The model under review builds one solid part; all positions refer to its coordinate system, in mm. Face numbers are marked on the shaded views. A direction names the side the tool comes from. Coordinates: 2 decimals unless noted, no trailing zeros. Write each loop counter-clockwise with the first axis right and the second up, starting at its lowest first coordinate (ties: lowest second). Pieces come first, ordered by that corner, then holes. Notation, with made-up numbers: M -15.5,3 L 12.5,3 A9 cw 12.5,15 Z; hole C 46.25,4.25 d6. An arc over 180 degrees is marked long. Answer as a JSON object with one key per item and string values.
```python
from build123d import *

# Parameters (mm, degrees)
SKETCH1_W                 = 32.5
SKETCH1_H                 = 42
BOSS_EXTRUDE2_DEPTH       = 5
F_2_56_TAPPED_HOLE1_D     = 1.778
F_2_56_TAPPED_HOLE1_DEPTH = 7.46583491
F_2_56_TAPPED_HOLE1_TIP   = 0.53416509
F_2_56_TAPPED_HOLE2_D     = 1.778
F_2_56_TAPPED_HOLE2_DEPTH = 7.46583491
F_2_56_TAPPED_HOLE2_TIP   = 0.53416509
CUT_EXTRUDE1_DEPTH        = 5
SKETCH10_W                = 10
SKETCH10_H                = 6.5
CUT_EXTRUDE2_DEPTH        = 2.5


with BuildPart() as part:
    # Sketch1 → Boss-Extrude2 (new body)
    with BuildSketch(Plane.XY):
        with Locations((16.25, 21)):
            Rectangle(SKETCH1_W, SKETCH1_H)
    extrude(amount=BOSS_EXTRUDE2_DEPTH)

    # #2-56 Tapped Hole1
    with Locations(Plane.ZY):
        with Locations((2.5, 34), (2.5, 8)):
            Hole(F_2_56_TAPPED_HOLE1_D / 2, depth=F_2_56_TAPPED_HOLE1_DEPTH)
            with Locations((0, 0, -(F_2_56_TAPPED_HOLE1_DEPTH + F_2_56_TAPPED_HOLE1_TIP / 2))):  # 118° drill point
                Cone(0, F_2_56_TAPPED_HOLE1_D / 2, F_2_56_TAPPED_HOLE1_TIP, mode=Mode.SUBTRACT)

    # #2-56 Tapped Hole2
    with Locations(Plane(origin=(32.5, 0, 0), x_dir=(0, 0, -1), z_dir=(1, 0, 0))):
        with Locations((-2.5, 34), (-2.5, 8)):
            Hole(F_2_56_TAPPED_HOLE2_D / 2, depth=F_2_56_TAPPED_HOLE2_DEPTH)
            with Locations((0, 0, -(F_2_56_TAPPED_HOLE2_DEPTH + F_2_56_TAPPED_HOLE2_TIP / 2))):  # 118° drill point
                Cone(0, F_2_56_TAPPED_HOLE2_D / 2, F_2_56_TAPPED_HOLE2_TIP, mode=Mode.SUBTRACT)

    # Sketch9 → Cut-Extrude1 (cut)
    with BuildSketch(Plane(origin=(0, 0, 0), x_dir=(-1, 0, 0), z_dir=(0, 0, -1))):
        with BuildLine():
            ThreePointArc((-15.1, 21), (-12.1, 18), (-9.1, 21))
            Line((-9.1, 21), (-12.1, 21))
            Line((-12.1, 21), (-15.1, 21))
        make_face()
        with BuildLine():
            Line((-12.1, 21), (-9.1, 21))
            ThreePointArc((-9.1, 21), (-12.1, 24), (-15.1, 21))
            Line((-15.1, 21), (-12.1, 21))
        make_face()
    extrude(amount=-CUT_EXTRUDE1_DEPTH, mode=Mode.SUBTRACT)

    # Sketch10 → Cut-Extrude2 (cut)
    with BuildSketch(Plane(origin=(0, 0, 0), x_dir=(-1, 0, 0), z_dir=(0, 0, -1))):
        with Locations((-16.25, 38.75)):
            Rectangle(SKETCH10_W, SKETCH10_H)
    extrude(amount=-CUT_EXTRUDE2_DEPTH, mode=Mode.SUBTRACT)


solid = part.part
```
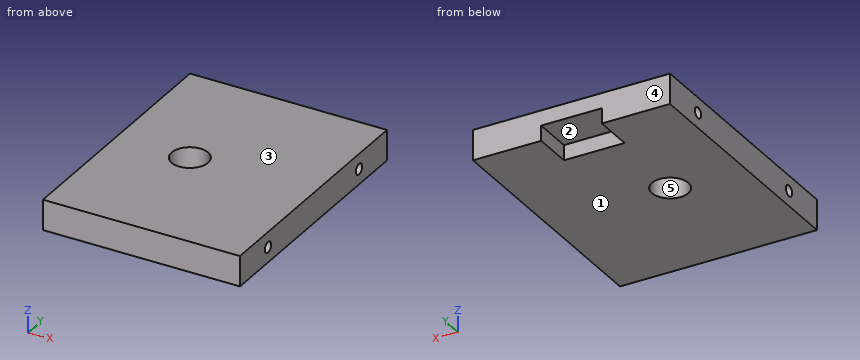
(1) Add section B-B on y = 36.5. Give the boundary of the cut face in (x, z).
Results list:
{"outline": "M 0,0 L 11.25,0 L 11.25,2.5 L 21.25,2.5 L 21.25,0 L 32.5,0 L 32.5,5 L 0,5 Z"}
(2) Add section C-C on x = 27.5. Give the boundary of the cut face in (y, z), and give its area (3 significant figures).
Results list:
{"outline": "M 0,0 L 42,0 L 42,5 L 0,5 Z; hole C 8,2.5 d1.78; hole C 34,2.5 d1.78", "area": "205 mm²"}
(3) Add section D-D on z = 4.1. Give the boundary of the cut face in (x, y).
Results list:
{"outline": "M 0,0 L 32.5,0 L 32.5,42 L 0,42 Z; hole C 12.1,21 d6"}
(4) Wall thickness on line 1 along Y through (x, z) = (28, 2.5); line 2 along X through (y, z) = (39.5, 2.4); line 3 along Y through (x, z) = (5.5, 2.85): over which ranges is each line inside the solid? List them lowest first. Write a range as from..to.
Results list:
{"line 1": "0..7.11, 8.89..33.11, 34.89..42", "line 2": "0..11.25, 21.25..32.5", "line 3": "0..7.18, 8.82..33.18, 34.82..42"}
(5) Add section A-A on x = 12.1. Give the boundary of the cut face in (y, z).
Results list:
{"outline": "M 0,0 L 18,0 L 18,5 L 0,5 Z; M 24,0 L 35.5,0 L 35.5,2.5 L 42,2.5 L 42,5 L 24,5 Z"}
(6) For pin 1 Ø3 at (y, z) = (34, 2.5) entering from -X; pin 2 Ø1.1 at (y, z) = (34, 2.5) entering from +X; pin 3 Ø5.5 at (x, y) = (12.1, 21) entering from +Z; pin 4 Ø0.8 at (x, z) = (18, 2) entering from +Y, all flat-tipped, find the tip position at first contact; note any pin that passes through.
Results list:
{"pin 1": "x = 0", "pin 2": "x = 24.83", "pin 3": "through", "pin 4": "y = 35.5"}
(7) Draft analysis for pull direction Y (two halves, no side actions). For the marked faces 3, 4 and 5, state which applies: released by +Y, released by -Y, zero draft, split by the parting line, or undercut.
Results list:
{"face 3": "zero draft", "face 4": "released by +Y", "face 5": "undercut"}
(8) For the marked faces 1 and 2, list the 3-axis set-ups (+Z, -Z, +X, -X, +Y, -Y) from which the entire face can be reached by the end or side of a thin tool; tool diameter is ignored.
Results list:
{"face 1": "-Z, +X, -X, +Y, -Y", "face 2": "-Z, +Y"}
